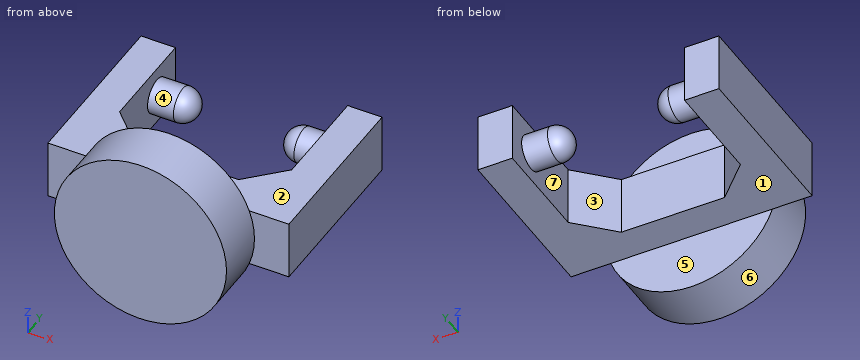
```python
from build123d import *

# Parameters (mm, degrees)
SKETCH1_R           = 12.5
BOSS_EXTRUDE1_DEPTH = 7.5
SKETCH2_W           = 35
SKETCH2_H           = 8.580767914
BOSS_EXTRUDE2_DEPTH = 25
SKETCH3_W           = 25
SKETCH3_H           = 8.580767914
CUT_EXTRUDE1_DEPTH  = 20
SKETCH4_R           = 2.5
BOSS_EXTRUDE3_DEPTH = 6.25
SKETCH5_R           = 2.5
BOSS_EXTRUDE4_DEPTH = 6.25
CHAMFER1_SIZE       = 5
CHAMFER2_SIZE       = 5
FILLET1_R           = 2.5
FILLET2_R           = 2.5


with BuildPart() as part:
    # Sketch1 → Boss-Extrude1 (new body)
    with BuildSketch(Plane(origin=(0, 0, 0), x_dir=(1, 0, 0), z_dir=(0, 1, 0))):
        Circle(SKETCH1_R)
    extrude(amount=BOSS_EXTRUDE1_DEPTH)

    # Sketch2 → Boss-Extrude2 (add)
    with BuildSketch(Plane(origin=(0, 7.5, 0), x_dir=(1, 0, 0), z_dir=(0, 1, 0))):
        Rectangle(SKETCH2_W, SKETCH2_H)
    extrude(amount=BOSS_EXTRUDE2_DEPTH)

    # Sketch3 → Cut-Extrude1 (cut)
    with BuildSketch(Plane(origin=(0, 32.5, 0), x_dir=(1, 0, 0), z_dir=(0, 1, 0))):
        Rectangle(SKETCH3_W, SKETCH3_H)
    extrude(amount=-CUT_EXTRUDE1_DEPTH, mode=Mode.SUBTRACT)

    # Sketch4 → Boss-Extrude3 (add)
    with BuildSketch(Plane(origin=(-12.5, 0, 0), x_dir=(0, 0, -1), z_dir=(1, 0, 0))):
        with Locations((0, 27.5)):
            Circle(SKETCH4_R)
    extrude(amount=BOSS_EXTRUDE3_DEPTH)

    # Sketch5 → Boss-Extrude4 (add)
    with BuildSketch(Plane.ZY.offset(-12.5)):
        with Locations((0, 27.5)):
            Circle(SKETCH5_R)
    extrude(amount=BOSS_EXTRUDE4_DEPTH)

    # Chamfer1
    chamfer1_edges = [part.edges().sort_by_distance(p)[0] for p in [
        (-12.5, 12.5, 0),
    ]]
    chamfer(chamfer1_edges, length=CHAMFER1_SIZE)

    # Chamfer2
    chamfer2_edges = [part.edges().sort_by_distance(p)[0] for p in [
        (12.5, 12.5, 0),
    ]]
    chamfer(chamfer2_edges, length=CHAMFER2_SIZE)

    # Fillet1
    fillet1_edges = [part.edges().sort_by_distance(p)[0] for p in [
        (-6.25, 27.5, 2.5),
    ]]
    fillet(fillet1_edges, radius=FILLET1_R)

    # Fillet2
    fillet2_edges = [part.edges().sort_by_distance(p)[0] for p in [
        (6.25, 27.5, -2.5),
    ]]
    fillet(fillet2_edges, radius=FILLET2_R)


solid = part.part
```
Geometry check sheet. Reference: the model listing, model coordinates, mm. Face numbers are marked on the shaded views. A direction names the side the tool comes from. Coordinates: 2 decimals unless noted, no trailing zeros. Order: outer loops, then holes, each group sorted by start corner. A loop starts at its lowest first (then second) coordinate and runs counter-clockwise, first axis right, second up. Notation, with made-up numbers: M 32.25,-26 L 78.25,-26 A13 ccw 78.25,-9 Z; hole C 28,-2.5 d4. An arc over 180 degrees is marked long. One line per question, with ' | ' between items. Start each with the question number.
Item 1: Cross-section at C-C on z = 0. Enter the section's corners in (x, y), then the cut area to 3 significant figures.
Item 2: Draft check along X on the marked faces 5, 6 and 7. Enter one of: pulls with the +X half, pulls with the -X half, needs draft (parallel to the pull), parting line crosses it, or undercut.
Item 3: Cross-section at A-A on y = 21. Enter the section's corners in (x, z).
Item 4: Set-up check for the marked faces 1, 2, 3 and 4: record each of +Z, -Z, +X, -X, +Y, -Y from which the full face is reachable in a straight line by a thin tool's end or side.
Item 5: Material ranges on L1, parallel to X at y = 20, z = -0.5; L2, parallel to Z at x = 16.5, y = 30; L3, parallel to Y at x = -5.5, z = 4, recorded low to high. Write a range as [from, to].
Item 6: Cross-section at B-B on x = -7. Enter the section's corners in (y, z), then the cut area to 3 significant figures.
Item 7: Gauge pin test, flat ends, axial feed: pin 1 (1.5 mm diameter, centred on x = 11, y = 9, fed in from -Z); pin 2 (2 mm diameter, centred on x = -10, z = -5, fed in from -Y); pin 3 (3 mm diameter, centred on x = -7.5, y = 12, fed in from +Z); pin 4 (2.5 mm diameter, centred on x = -2.5, z = 8.5, fed in from +Y). Record the tip position at first contact, or that the pin passes through.
Item 8: Cross-section at D-D on x = 0. Enter the section's corners in (y, z).
Findings:
1) outline: M -17.5,7.5 L -12.5,7.5 L -12.5,0 L 12.5,0 L 12.5,7.5 L 17.5,7.5 L 17.5,32.5 L 12.5,32.5 L 12.5,30 L 8.75,30 A2.5 ccw 8.75,25 L 12.5,25 L 12.5,17.5 L 7.5,12.5 L -7.5,12.5 L -12.5,17.5 L -12.5,25 L -8.75,25 A2.5 ccw -8.75,30 L -12.5,30 L -12.5,32.5 L -17.5,32.5 Z | area: 645 mm²
2) face 5: needs draft | face 6: parting line crosses it | face 7: undercut
3) outline: M -17.5,-4.29 L -12.5,-4.29 L -12.5,4.29 L -17.5,4.29 Z; M 12.5,-4.29 L 17.5,-4.29 L 17.5,4.29 L 12.5,4.29 Z
4) face 1: -Z, +X, -X, +Y | face 2: +Z, +X, -X, +Y | face 3: +Z, -Z | face 4: none
5) L1: x = [-17.5, -12.5], [12.5, 17.5] | L2: z = [-4.29, 4.29] | L3: y = [0, 12.5]
6) outline: M 0,-10.36 L 7.5,-10.36 L 7.5,-4.29 L 12.5,-4.29 L 12.5,4.29 L 7.5,4.29 L 7.5,10.36 L 0,10.36 Z; C 27.5,0 d3.57 | area: 208 mm²
7) pin 1: stops at z = -4.29 | pin 2: stops at y = 0 | pin 3: stops at z = 4.29 | pin 4: stops at y = 7.5
8) outline: M 0,-12.5 L 7.5,-12.5 L 7.5,-4.29 L 12.5,-4.29 L 12.5,4.29 L 7.5,4.29 L 7.5,12.5 L 0,12.5 Z
